Autodesk Inventor part; units mm, degrees
ref_plane "YZ Plane" through (0, 0, 0) normal (1, 0, 0) x (0, 1, 0)
ref_plane "XZ Plane" through (0, 0, 0) normal (0, 1, 0) x (-1, 0, 0)
ref_plane "XY Plane" through (0, 0, 0) normal (0, 0, 1) x (1, 0, 0)
sketch "Sketch1" plane through (0, 0, 0) normal (1, 0, 0) x (0, 1, 0)
  point P0 (0, 0)
sketch "Sketch2" plane through (0, 0, 0) normal (1, 0, 0) x (0, 1, 0)
  line L0 (-127.5, -112) -> (127.5, -112)
  line L1 (127.5, -112) -> (127.5, 112)
  line L2 (127.5, 112) -> (-127.5, 112)
  line L3 (-127.5, 112) -> (-127.5, -112)
  line L4 (-127.5, -112) -> (127.5, 112) construction
  line L5 (127.5, -112) -> (-127.5, 112) construction
  line L6 (127.5, -52) -> (92.5, -112)
  point P0 (0, 0)
  dimension "d0" = 255
  dimension "d1" = 224
  dimension "d2" = 35
  dimension "d3" = 60
extrude "Extrusion1" add sketch "Sketch2" along normal blind 500 contours L3 L2 L1 L6 L0
shell "Shell1" thickness 22.5 removed faces 0
ref_plane "Work Plane1" through (0, -127.5, -100.75) normal (0, 0, -1) x (-1, 0, 0)
sketch "Sketch3" plane through (0, -127.5, -112) normal (0, 0, -1) x (-1, 0, 0)
  line L0 (-105.6, 103) -> (-190.4, 103)
  line L1 (-190.4, 103) -> (-190.4, 129.4)
  line L2 (-190.4, 129.4) -> (-105.6, 129.4)
  line L3 (-105.6, 129.4) -> (-105.6, 103)
  point P0 (0, 127.5)
  dimension "d7" = 84.8
  dimension "d8" = 26.4
extrude "Extrusion2" cut sketch "Sketch3" against normal blind 201.5
sketch "Sketch4" plane through (0, -127.5, -112) normal (0, 0, -1) x (-1, 0, 0)
  line L0 (-269.6, 140.8) -> (-320.36, 140.8)
  line L1 (-320.36, 140.8) -> (-320.36, 90.04)
  line L2 (-320.36, 90.04) -> (-269.6, 90.04)
  line L3 (-269.6, 90.04) -> (-269.6, 140.8)
  line L4 (0, 220) -> (-500, 220)
  line L5 (-190.4, 103) -> (-190.4, 129.4)
  point P0 (0, 127.5)
  dimension "d11" = 50.76
  dimension "d12" = 50.76
  dimension "d13" = 79.2
  dimension "d14" = 79.2
extrude "Extrusion3" cut sketch "Sketch4" against normal blind 201.5
Model file for the job. Use its own axes, mm. A direction names the side the tool comes from. Give positions to 0.01 mm unless a question says otherwise; leave off trailing zeros. Order: outer loops, then holes, each group sorted by start corner. A loop starts at its lowest first (then second) coordinate and runs counter-clockwise, first axis right, second up. Notation, with made-up numbers: (-15, 36.25) - (6, 36.25) arc R17 ccw to (6, 55.25) - close; hole circle Ø10 at (-16, 5). An arc over 180 degrees is marked (long way). One line per item, written item: value.
Item 1: Slice it at A-A (x = 216.5). List the corners of the cut face in (y, z), then the cut area to 3 significant figures.
Response values:
outline: (-127.5, -112) - (92.5, -112) - (127.5, -52) - (127.5, 112) - (-127.5, 112) - close; hole (-105, -89.5) - (79.58, -89.5) - (105, -45.92) - (105, 89.5) - (-105, 89.5) - close
area: 19,000 mm2
Item 2: Tool access for faces 5 (the flat face through (247, -105, 1)), 6 (the flat face through (269.6, -12, -101)), 7 (the flat face through (246, -127.5, 2)): list every direction of +Z, -Z, +X, -X, +Y, -Y with a clear straight run to the whole face (end or side of a thin tool).
Response values:
face 5: none
face 6: -Z
face 7: +Z, -Z, +X, -X, -Y
Item 3: Slice it at B-B (y = 53). List the corners of the cut face in (x, z).
Response values:
outline: (0, -112) - (500, -112) - (500, 112) - (0, 112) - close; hole (22.5, -89.5) - (477.5, -89.5) - (477.5, 89.5) - (22.5, 89.5) - close
Item 4: Pin check, flat tips, straight feed: pin 1 Ø18 at (x, z) = (303.5, -98.5) entering from +Y (3 decimals); pin 2 Ø18 at (x, z) = (161.5, -99.5) entering from +Y. Stop position of each tip, or through.
Response values:
pin 1: y = 105.625
pin 2: y = 105.04
Item 5: Slice it at D-D (x = 290). List the corners of the cut face in (y, z), then the cut area to 3 significant figures.
Response values:
outline: (-127.5, -112) - (-37.46, -112) - (-37.46, -89.5) - (-105, -89.5) - (-105, 89.5) - (105, 89.5) - (105, -45.92) - (79.58, -89.5) - (13.3, -89.5) - (13.3, -112) - (92.5, -112) - (127.5, -52) - (127.5, 112) - (-127.5, 112) - close
area: 17,900 mm2
Item 6: Slice it at C-C (z = -34.5). List the corners of the cut face in (x, y), then the cut area to 4 significant figures.
Response values:
outline: (0, -127.5) - (500, -127.5) - (500, 127.5) - (0, 127.5) - close; hole (22.5, -105) - (477.5, -105) - (477.5, 105) - (22.5, 105) - close
area: 31,950 mm2
Item 7: Two-plate mould, pull along X, no slides. Class faces 1 (the flat face through (0, -2, 2)), 2 (the flat face through (320.36, -12, -101)), 3 (the flat face through (105.6, -11, -101)), 4 (the flat face through (246, -19, -112)): released by +X, released by -X, zero draft, split by the parting line, or undercut.
Response values:
face 1: released by -X
face 2: undercut
face 3: undercut
face 4: zero draft
Item 8: Wall check: line 1 (Y direction, x = 375.5, z = 25); line 2 (Z direction, x = 309.5, y = 15.5); line 3 (X direction, y = -33.5, z = -54.5). Give the ranges that are in metal, low to high.
Response values:
line 1: -127.5 to -105, 105 to 127.5
line 2: -112 to -89.5, 89.5 to 112
line 3: 0 to 22.5, 477.5 to 500
